Could you check a few things on this model? Use its own coordinates, in mm. A direction names the side the tool comes from. Give positions to 0.01 mm unless a question says otherwise; leave off trailing zeros. Write each loop counter-clockwise with the first axis right and the second up, starting at its lowest first coordinate (ties: lowest second). Pieces come first, ordered by that corner, then holes. Notation, with made-up numbers: M -18,18 L -6,18 A20 ccw -6,30 Z; hole C 72.5,-40 d9. An arc over 180 degrees is marked long. One line per item, written item: value.
```python
from build123d import *

# Parameters (mm, degrees)
ESQUISSE1_R             = 2
BOSS_EXTRU_1_DEPTH      = 66
ESQUISSE2_W             = 7.5
ESQUISSE2_H             = 2
ENL_V_MAT_EXTRU_1_DEPTH = 2
ESQUISSE3_W             = 7.5
ESQUISSE3_H             = 2
ENL_V_MAT_EXTRU_2_DEPTH = 2


with BuildPart() as part:
    # Esquisse1 → Boss.-Extru.1 (new body)
    with BuildSketch(Plane.XY):
        Circle(ESQUISSE1_R)
    extrude(amount=BOSS_EXTRU_1_DEPTH)

    # Esquisse2 → Enlèv. mat.-Extru.1 (cut)
    with BuildSketch(Plane.XY.offset(66)):
        Rectangle(ESQUISSE2_W, ESQUISSE2_H)
    extrude(amount=-ENL_V_MAT_EXTRU_1_DEPTH, mode=Mode.SUBTRACT)

    # Esquisse3 → Enlèv. mat.-Extru.2 (cut)
    with BuildSketch(Plane(origin=(0, 0, 0), x_dir=(-1, 0, 0), z_dir=(0, 0, -1))):
        Rectangle(ESQUISSE3_W, ESQUISSE3_H)
    extrude(amount=-ENL_V_MAT_EXTRU_2_DEPTH, mode=Mode.SUBTRACT)


solid = part.part
```
1) On a 3-axis mill with a long thin cutter (end or side, diameter ignored), from which of +Z, -Z, +X, -X, +Y, -Y can I reach the whole of each face in a straight line? I mean faces 4 (the face through (0, 1.4, 0)), 5 (the face through (0, 1, 65)), 6 (the face through (0, -1, 1)). Say none if no direction works.
Outcome:
face 4: -Z, +X, -X, +Y, -Y
face 5: +Z, +X, -X
face 6: -Z, +X, -X
2) If we section it at A-A, the plane x = -1.2: Write out the boundary of the cut face in (y, z).
Outcome:
outline: M -1.6,0 L -1,0 L -1,2 L 1,2 L 1,0 L 1.6,0 L 1.6,66 L 1,66 L 1,64 L -1,64 L -1,66 L -1.6,66 Z
3) If we section it at C-C, the plane y = 0: Write out the boundary of the cut face in (x, z).
Outcome:
outline: M -2,2 L 2,2 L 2,64 L -2,64 Z
4) If we section it at B-B, the plane z = 61: Write out the boundary of the cut face in (x, y).
Outcome:
outline: C 0,0 d4
5) Please list where these lines run through material, in increasing order: L1, parallel to Z at x = -1.1, y = -0.25; L2, parallel to Y at x = 1, z = 44; L3, parallel to X at y = 0.95, z = 8. Write a range as from..to.
Outcome:
L1: z = 2..64
L2: y = -1.73..1.73
L3: x = -1.76..1.76
6) I'm going to push flat-ended pins straight in: pin 1 (0.6 mm diameter, centred on x = 0.5, z = 0.5, fed in from -Y); pin 2 (1.6 mm diameter, centred on x = -1, y = 0, fed in from +Z). Where does each tip first touch, or does it pass through?
Outcome:
pin 1: stops at y = -1.99
pin 2: stops at z = 64
7) We'd pull the mould along Y, two halves only. Please class faces 1 (the face through (0, -2, 33)), 2 (the face through (0, 1.4, 66)), 3 (the face through (0, 0, 64)): pulls with the +Y half, pulls with the -Y half, needs draft (parallel to the pull), parting line crosses it, or undercut.
Outcome:
face 1: parting line crosses it
face 2: needs draft
face 3: undercut
